from build123d import *

# Parameters (mm, degrees)
SKETCH_1_W      = 2
SKETCH_1_H      = 2
EXTRUDE_1_DEPTH = 12
SKETCH_2_R      = 1
EXTRUDE_2_DEPTH = 3
EXTRUDE_START   = 3
SKETCH_3_R      = 1
EXTRUDE_3_DEPTH = 3


with BuildPart() as part:
    # Эскиз1 → Бобышка-Вытянуть1 (new body)
    with BuildSketch(Plane.XY):
        Rectangle(SKETCH_1_W, SKETCH_1_H)
    extrude(amount=EXTRUDE_1_DEPTH)

    # Эскиз2 → Бобышка-Вытянуть2 (add)
    with BuildSketch(Plane.XY.offset(12)):
        Circle(SKETCH_2_R)
    extrude(amount=EXTRUDE_2_DEPTH)

    # Эскиз3 → Бобышка-Вытянуть3 (add)
    with BuildSketch(Plane(origin=(0, 0, 0), x_dir=(-1, 0, 0), z_dir=(0, 0, -1)).offset(EXTRUDE_START)):
        with Locations(Location((0, 0, 0), (0, 0, 180))):
            Circle(SKETCH_3_R)
    extrude(amount=-EXTRUDE_3_DEPTH)


solid = part.part
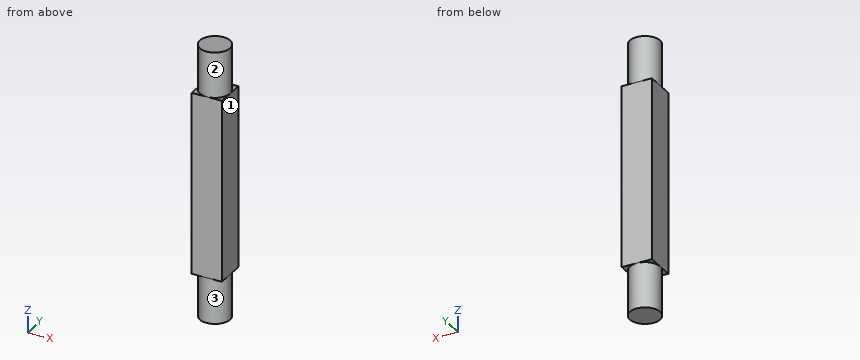
Could you check a few things on this model? Use its own coordinates, in mm. Face numbers are marked on the shaded views. A direction names the side the tool comes from. Round coordinates to 2 decimals unless told otherwise and drop trailing zeros. Write each loop counter-clockwise with the first axis right and the second up, starting at its lowest first coordinate (ties: lowest second). Pieces come first, ordered by that corner, then holes. Notation, with made-up numbers: (72, -20.5) - (98, -20.5) arc R31 ccw to (98, 13.5) - close; hole circle Ø7 at (66, 12.5). An arc over 180 degrees is marked (long way). Put each result on its own line as item: value. Start each with the question number.
(1) I need wall thicknesses on probe 1 along X at (y, z) = (-0.2, -1); probe 2 along Y at (x, z) = (0.85, -0.5). Which ranges of each line are inside material? Lowest first, please.
(2) I want a section at B-B, the plane z = -0.75. Please give me the cut outline in (x, y).
(3) For the marked faces 1, 2 and 3, which set-ups out of +Z, -Z, +X, -X, +Y, -Y let a thin tool reach every point of the face, with its end or its side?
(4) I want a section at C-C, the plane x = 0.5. Please give me the cut outline in (y, z).
(5) I want a section at A-A, the plane x = -0.6. Please give me the cut outline in (y, z), plus the area to 3 significant figures.
Here are the results:
1. probe 1: x = -0.98 to 0.98
1. probe 2: y = -0.53 to 0.53
2. outline: circle Ø2 at (0, 0)
3. face 1: +Z, -Z, +X, +Y, -Y
3. face 2: +Z
3. face 3: -Z
4. outline: (-1, 0) - (-0.87, 0) - (-0.87, -3) - (0.87, -3) - (0.87, 0) - (1, 0) - (1, 12) - (0.87, 12) - (0.87, 15) - (-0.87, 15) - (-0.87, 12) - (-1, 12) - close
5. outline: (-1, 0) - (-0.8, 0) - (-0.8, -3) - (0.8, -3) - (0.8, 0) - (1, 0) - (1, 12) - (0.8, 12) - (0.8, 15) - (-0.8, 15) - (-0.8, 12) - (-1, 12) - close
5. area: 33.6 mm^2
